The figure shows three views and two pictorial views of one solid part (mm, origin at its lowest corner). Answer the questions. Round coordinates to 2 decimals unless told otherwise and drop trailing zeros. Write each loop counter-clockwise with the first axis right and the second up, starting at its lowest first coordinate (ties: lowest second). Pieces come first, ordered by that corner, then holes.
Item 1: For a pull along X with two mould halves and no side action, classify the marked faces 1, 2 and 3 as +X half, -X half, draft (parallel to the pull), parting line (faces both ways), or undercut.
Item 2: Each of these flat-tipped pins is pushed along its axis until it touches: pin 1 (0.5 mm diameter, centred on x = 59.5, y = 25, fed in from -Z); pin 2 (10 mm diameter, centred on x = 10.5, z = 7.5, fed in from +Y); pin 3 (1.1 mm diameter, centred on x = 17.5, z = 40.5, fed in from +Y); pin 4 (0.8 mm diameter, centred on x = 0.5, y = 26.5, fed in from +Z). Where does it stop, or does it pass through?
Item 3: Find section B-B on z = 37.5. Give the vertices of the cut face in (x, y) (1 decimal).
Item 4: Find section A-A on y = 50. Give the vertices of the cut face in (x, z) (1 decimal).
Item 5: Find section D-D on x = 47. Give the vertices of the cut face in (y, z).
Item 6: Find the intervals of material crossed by probe 1 along X at (y, z) = (59, 6); probe 2 along Z at (x, y) = (34, 43); probe 3 along Y at (x, z) = (59.85, 10) (1 decimal), in increasing order.
Item 7: Find section C-C on z = 10. Give the vertices of the cut face in (x, y) (1 decimal).
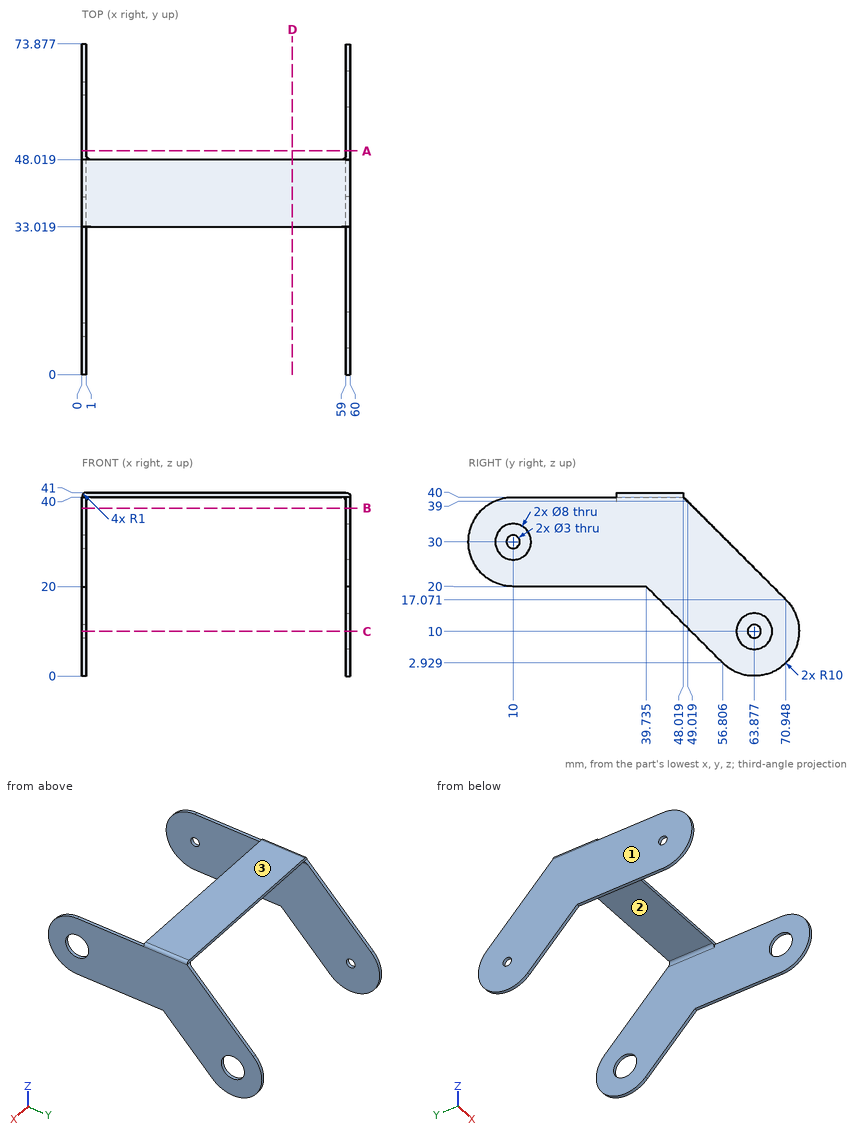
Check values:
1. face 1: -X half
1. face 2: undercut
1. face 3: draft
2. pin 1: stops at z = 20
2. pin 2: passes through
2. pin 3: stops at y = 48.02
2. pin 4: stops at z = 40
3. outline: (0, 3.4) - (1, 3.4) - (1, 50.5) - (0, 50.5) - close; (59, 3.4) - (60, 3.4) - (60, 50.5) - (59, 50.5) - close
4. outline: (0, 9.7) - (1, 9.7) - (1, 38) - (0, 38) - close; (59, 9.7) - (60, 9.7) - (60, 38) - (59, 38) - close
5. outline: (33.02, 40) - (48.02, 40) - (48.02, 41) - (33.02, 41) - close
6. probe 1: x = 0 to 1, 59 to 60
6. probe 2: z = 40 to 41
6. probe 3: y = 49.7 to 59.9, 67.9 to 73.9
7. outline: (0, 49.7) - (1, 49.7) - (1, 62.4) - (0, 62.4) - close; (0, 65.4) - (1, 65.4) - (1, 73.9) - (0, 73.9) - close; (59, 49.7) - (60, 49.7) - (60, 59.9) - (59, 59.9) - close; (59, 67.9) - (60, 67.9) - (60, 73.9) - (59, 73.9) - close
